Verification items for the finished model (mm, model axes). Face numbers are marked on the shaded views. A direction names the side the tool comes from. Coordinates: 2 decimals unless noted, no trailing zeros. Loops run counter-clockwise (first coordinate to the right, second up) from the corner with the lowest first, then second, coordinate; pieces in that order, holes last. Notation, with made-up numbers: (-5.5, -37.75) -> (17.5, -37.75) arc R15 cw to (17.5, -17.75) -> close; hole circle Ø6 at (-14.75, -28). An arc over 180 degrees is marked (long way). Use CSV: the item, a comma, the result in double quotes. Start each with the question number.
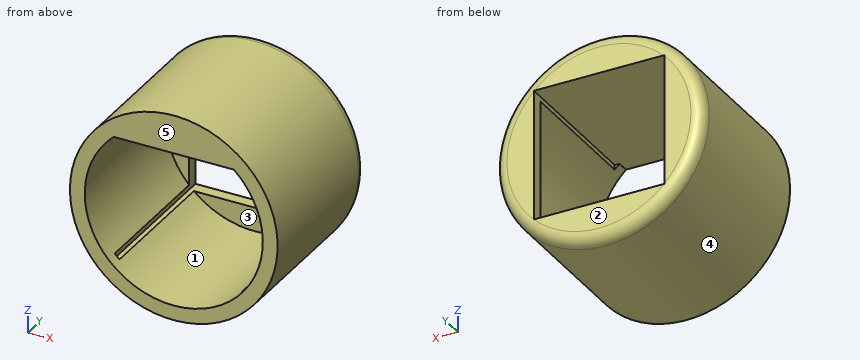
Autodesk Inventor part; units mm, degrees
ref_plane "YZ Plane" through (0, 0, 0) normal (1, 0, 0) x (0, 1, 0)
ref_plane "XZ Plane" through (0, 0, 0) normal (0, 1, 0) x (-1, 0, 0)
ref_plane "XY Plane" through (0, 0, 0) normal (0, 0, 1) x (1, 0, 0)
sketch "Sketch1" plane through (0, 0, 0) normal (0, 1, 0) x (-1, 0, 0)
  circle A0 centre (0, 0) radius 22.225
  dimension "d0" = 44.45
extrude "Extrusion1" add sketch "Sketch1" along normal blind 34.29
fillet "Fillet1" radius 2.54 1 edges at (22.225, 34.29, 0)
sketch "Sketch2" plane through (0, 0, 0) normal (0, -1, 0) x (1, 0, 0)
  circle A0 centre (0, 0) radius 19.05
  dimension "d4" = 38.1
extrude "Extrusion2" cut sketch "Sketch2" against normal blind 31.75
sketch "Sketch3" plane through (0, 34.29, 0) normal (0, 1, 0) x (1, 0, 0)
  line L0 (0, 0) -> (0, -13.97)
  line L1 (0, 0) -> (-13.97, 0)
  line L2 (-14.0204, -14.0204) -> (13.9196, -14.0204)
  line L3 (13.9196, -14.0204) -> (13.9196, 13.9196)
  line L4 (13.9196, 13.9196) -> (-14.0204, 13.9196)
  line L5 (-14.0204, 13.9196) -> (-14.0204, -14.0204)
  dimension "d7" = 13.97
  dimension "d8" = 13.97
  dimension "d9" = 27.94
  dimension "d10" = 27.94
extrude "Extrusion3" cut sketch "Sketch3" against normal blind 31.75
sketch "Sketch4" plane through (0, 0, 0) normal (0, -1, 0) x (1, 0, 0)
  line L0 (13.8176, 14.0204) -> (-13.8176, 14.0204)
  line L1 (0, 14.0204) -> (-12.8969, 14.0204)
  arc A0 (13.9196, -13.0057) -> (13.9196, 13.0057) centre (0, 0) ccw
  line L2 (0, 14.0204) -> (12.8969, 14.0204)
  circle A1 centre (0, 0) radius 19.05
  point P0 (10.16, 10.16)
  point P1 (-10.16, 10.16)
  point P2 (12.8969, 14.0204)
  point P3 (-12.8969, 14.0204)
  point P4 (-13.8176, 14.0204)
extrude "Extrusion4" add sketch "Sketch4" against normal blind 34.29 contours L0 A1
properties part number "module" material "ABS Plastic"
1. Cross-section at A-A, the plane x = 0. Record the boundary of the cut face in (y, z) (3 decimals).
2. Cross-section at B-B, the plane z = 0. Record the boundary of the cut face in (x, y) (3 decimals).
3. Scan lines: line 1 (Z direction, x = 0, y = 15.5) (3 decimals); line 2 (Z direction, x = 8, y = 9.5); line 3 (X direction, y = 17, z = 5.5). Record each from-to range of solid material in increasing order.
4. Set-up check for the marked faces 1 and 2: record each of +Z, -Z, +X, -X, +Y, -Y from which the full face is reachable in a straight line by a thin tool's end or side.
5. Release check for a two-part mould opening along Z. For the marked faces 3, 4 and 5 record: released by +Z, released by -Z, zero draft, split by the parting line, or undercut.
6. Depth check by flat-ended pin: pin 1 (2.5 mm diameter, centred on x = 16.5, z = 5, fed in from -Y); pin 2 (8 mm diameter, centred on y = 6, z = -15.5, fed in from +X); pin 3 (3 mm diameter, centred on y = 6.5, z = 17.5, fed in from +X). Enter the tip coordinate at first touch or a pass-through.
Solution:
1,outline,"(0, -22.225) -> (31.75, -22.225) arc R2.54 ccw to (34.29, -19.685) -> (34.29, -13.92) -> (31.75, -13.92) -> (31.75, -19.05) -> (0, -19.05) -> close; (0, 14.02) -> (34.29, 14.02) -> (34.29, 19.685) arc R2.54 ccw to (31.75, 22.225) -> (0, 22.225) -> close"
2,outline,"(-22.225, 0) -> (-19.05, 0) -> (-19.05, 31.75) -> (-14.02, 31.75) -> (-14.02, 34.29) -> (-19.685, 34.29) arc R2.54 ccw to (-22.225, 31.75) -> close; (13.92, 31.75) -> (19.05, 31.75) -> (19.05, 0) -> (22.225, 0) -> (22.225, 31.75) arc R2.54 ccw to (19.685, 34.29) -> (13.92, 34.29) -> close"
3,line 1,"z = -22.225 to -19.05, 14.02 to 22.225"
3,line 2,"z = -20.74 to -17.29, 14.02 to 20.74"
3,line 3,"x = -21.53 to -18.24, 18.24 to 21.53"
4,face 1,"-Y"
4,face 2,"+Z, -Z, +X, -X, +Y"
5,face 3,"undercut"
5,face 4,"split by the parting line"
5,face 5,"zero draft"
6,pin 1,"stops at y = 31.75"
6,pin 2,"stops at x = 19.02"
6,pin 3,"stops at x = 15.43"
